Can you work these out from the model? Positions are in its coordinate system, mm. A direction names the side the tool comes from. Give positions to 0.01 mm unless a question says otherwise; leave off trailing zeros. Loops run counter-clockwise (first coordinate to the right, second up) from the corner with the lowest first, then second, coordinate; pieces in that order, holes last. Notation, with made-up numbers: M 72,37 L 115,37 A28 cw 115,55 Z; hole C 68,82.25 d2. An arc over 180 degrees is marked long. Use CSV: the item, a comma, the result in double quotes.
from build123d import *

# Parameters (mm, degrees)
SKETCH1_R           = 6.5
BOSS_EXTRUDE1_DEPTH = 15
BOSS_EXTRUDE3_DEPTH = 30
CUT_EXTRUDE1_DEPTH  = 10


with BuildPart() as part:
    # Sketch1 → Boss-Extrude1 (new body)
    with BuildSketch(Plane(origin=(0, 0, 0), x_dir=(1, 0, 0), z_dir=(0, 1, 0))):
        Polygon((45, 30), (26.24355653, -40), (0, -40), (0, 0), (-35, 0), (-35, 30), align=None)
        with Locations((-20, 15)):
            Circle(SKETCH1_R, mode=Mode.SUBTRACT)
    extrude(amount=BOSS_EXTRUDE1_DEPTH)

    # Sketch5 → Boss-Extrude3 (add)
    with BuildSketch(Plane.XZ):
        Polygon((18.24355653, 40), (37, -30), (45, -30), (26.24355653, 40), align=None)
    extrude(amount=BOSS_EXTRUDE3_DEPTH)

    # Sketch7 → Cut-Extrude1 (cut)
    with BuildSketch(Plane(origin=(34.485571585, 0, 9.240381057), x_dir=(0.258819045, 0, -0.965925826), z_dir=(0.965925826, 0, 0.258819045))):
        with BuildLine():
            Line((-16.84470081, -8), (25.624631818, -8))
            ThreePointArc((25.624631818, -8), (31.624631818, -14), (25.624631818, -20))
            Line((25.624631818, -20), (-16.84470081, -20))
            ThreePointArc((-16.84470081, -20), (-22.84470081, -14), (-16.84470081, -8))
        make_face()
    extrude(amount=-CUT_EXTRUDE1_DEPTH, mode=Mode.SUBTRACT)


solid = part.part
Q1. I want a section at A-A, the plane x = -20. Please give me the cut outline in (y, z), then the cut area to 3 significant figures.
Model answer:
outline,"M 0,-30 L 15,-30 L 15,-21.5 L 0,-21.5 Z; M 0,-8.5 L 15,-8.5 L 15,0 L 0,0 Z"
area,"255 mm2"
Q2. I want a section at C-C, the plane z = -11. Please give me the cut outline in (x, y), then the cut area to 3 significant figures.
Model answer:
outline,"M -35,0 L -25.12,0 L -25.12,15 L -35,15 Z; M -14.88,0 L 31.91,0 L 31.91,-8 L 39.91,-8 L 39.91,15 L -14.88,15 Z; M 31.91,-30 L 39.91,-30 L 39.91,-20 L 31.91,-20 Z"
area,"1,110 mm2"
Q3. I want a section at B-B, the plane y = 6.5. Please give me the cut outline in (x, z), then the cut area to 3 significant figures.
Model answer:
outline,"M -35,-30 L 45,-30 L 26.24,40 L 0,40 L 0,0 L -35,0 Z; hole C -20,-15 d13"
area,"3,410 mm2"
Q4. If we mould it in two halves opening along X, with no side actions, what happens to faces 4 (the flat face through (-35, 7, -15)), 5 (the flat face through (13, 3, -30)), 6 (the cylindrical face through (-26.494, 7.395, -15.286)), 7 (the cylindrical face through (24.89, -14.13, 30.32))? For each: released by +X, released by -X, zero draft, split by the parting line, or undercut.
Model answer:
face 4,"released by -X"
face 5,"zero draft"
face 6,"undercut"
face 7,"released by +X"
Q5. Please list where these lines run through material, in increasing order: L1, parallel to Y at x = 35.5, z = 1; L2, parallel to Z at x = -20, y = 7; L3, parallel to Y at x = 16, z = 35. Write a range as from..to.
Model answer:
L1,"-30..-20, -8..15"
L2,"-30..-21.5, -8.5..0"
L3,"0..15"
Q6. I want a section at D-D, the plane y = -12. Please give me the cut outline in (x, z), then the cut area to 3 significant figures.
Model answer:
outline,"M 18.24,40 L 21.2,28.98 L 28.66,30.98 L 26.24,40 Z; M 35.12,-22.98 L 37,-30 L 45,-30 L 42.58,-20.98 Z"
area,"144 mm2"
Q7. For faces 1 (the flat face through (0, 7, 20)), 2 (the flat face through (19, -2, 40)), 3 (the flat face through (2, 0, -3)), which set-ups out of +Z, -Z, +X, -X, +Y, -Y let a thin tool reach every point of the face, with its end or its side?
Model answer:
face 1,"+Z, -X, +Y, -Y"
face 2,"+Z, +X, -X, +Y, -Y"
face 3,"-Z, -X, -Y"
Q8. I'm going to push flat-ended pins straight in: P1, Ø1.5, axis at y = 8, z = 29, coming from the -X side; P2, Ø1, axis at y = -21.5, z = -18.5, coming from the -X side; P3, Ø8, axis at y = -3, z = 21, coming from the +X side. Where does each tip first touch, or does it pass through?
Model answer:
P1,"x = 0"
P2,"x = 33.78"
P3,"x = 32.41"
